Source: CAD feature listing. Evaluate the final solid. Frame: model axes, mm. Face numbers are marked on the shaded views. Round coordinates to 2 decimals unless told otherwise and drop trailing zeros. Write each loop counter-clockwise with the first axis right and the second up, starting at its lowest first coordinate (ties: lowest second). Pieces come first, ordered by that corner, then holes. Notation, with made-up numbers: M -4.75,-13 L 47.25,-13 A17 cw 47.25,4 Z; hole C 89,49.5 d3. An arc over 180 degrees is marked long. Answer in a Markdown table with one row per item. Add a question column.
Item 1: Cut plane A-A on y = -0.3. Return loops of the section in (x, z), and give its area (3 significant figures).
Item 2: Material intervals for probe 1 along X at (y, z) = (0, 0.95); probe 2 along X at (y, z) = (-0.3, 0.5); probe 3 along Z at (x, y) = (-5.5, -0.35), sorted ascending.
Item 3: Mould query, pull axis Y, two halves, no side actions, for the marked faces 1, 2 and 3. Classes: released by +Y, released by -Y, zero draft, split by the parting line, or undercut.
Item 4: Cut plane B-B on z = 1.7. Return loops of the section in (x, y), and give its area (3 significant figures).
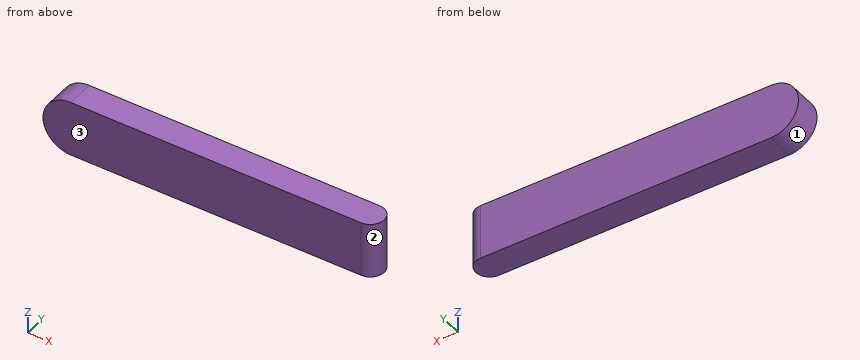
from build123d import *

# Parameters (mm, degrees)
SKETCH1_W           = 12
SKETCH1_H           = 1
BOSS_EXTRUDE1_DEPTH = 2
FILLET1_RADIUS      = 1
FILLET1_LENGTH      = 1
FILLET2_RADIUS      = 0.5
FILLET2_LENGTH      = 2


with BuildPart() as part:
    # Sketch1 → Boss-Extrude1 (new body)
    with BuildSketch(Plane.XY):
        Rectangle(SKETCH1_W, SKETCH1_H)
    extrude(amount=BOSS_EXTRUDE1_DEPTH)

    # Fillet1: full round fillet: the end face becomes a half cylinder, R = half its width
    fillet1_face = Plane((-6, 0, 1), x_dir=(0, 1, 0), z_dir=(-1, 0, 0))  # on the end face: x along it, z out of the body
    fillet1_slab = fillet1_face.offset(-FILLET1_RADIUS / 2) * Box(FILLET1_LENGTH, 2 * FILLET1_RADIUS, FILLET1_RADIUS, mode=Mode.PRIVATE)  # the body's end, R deep
    fillet1_round = Plane((-5, 0, 1), x_dir=(-1, 0, 0), z_dir=(0, 1, 0)) * Cylinder(FILLET1_RADIUS, FILLET1_LENGTH, mode=Mode.PRIVATE)  # its axis R under the face
    add(fillet1_slab - fillet1_round, mode=Mode.SUBTRACT)

    # Fillet2: full round fillet: the end face becomes a half cylinder, R = half its width
    fillet2_face = Plane((6, 0, 1), x_dir=(0, 0, 1), z_dir=(1, 0, 0))  # on the end face: x along it, z out of the body
    fillet2_slab = fillet2_face.offset(-FILLET2_RADIUS / 2) * Box(FILLET2_LENGTH, 2 * FILLET2_RADIUS, FILLET2_RADIUS, mode=Mode.PRIVATE)  # the body's end, R deep
    fillet2_round = Plane((5.5, 0, 1), x_dir=(1, 0, 0), z_dir=(0, 0, 1)) * Cylinder(FILLET2_RADIUS, FILLET2_LENGTH, mode=Mode.PRIVATE)  # its axis R under the face
    add(fillet2_slab - fillet2_round, mode=Mode.SUBTRACT)


solid = part.part
Results below:
| question | item | result |
|---|---|---|
| 1 | outline | M -5,0 L 5.9,0 L 5.9,2 L -5,2 A1 ccw Z |
| 1 | area | 23.4 mm2 |
| 2 | probe 1 | -6 to 6 |
| 2 | probe 2 | -5.87 to 5.9 |
| 2 | probe 3 | 0.13 to 1.87 |
| 3 | face 1 | zero draft |
| 3 | face 2 | split by the parting line |
| 3 | face 3 | released by -Y |
| 4 | outline | M -5.71,-0.5 L 5.5,-0.5 A0.5 ccw 5.5,0.5 L -5.71,0.5 Z |
| 4 | area | 11.6 mm2 |
